Work out the finished part from the listing and answer in its coordinate system (mm). Face numbers are marked on the shaded views. Give positions to 0.01 mm unless a question says otherwise; leave off trailing zeros. Write each loop counter-clockwise with the first axis right and the second up, starting at its lowest first coordinate (ties: lowest second). Pieces come first, ordered by that corner, then holes. Notation, with made-up numbers: (52.25, 42.25) - (98.25, 42.25) arc R20 cw to (98.25, 55.25) - close; hole circle Ø10 at (46.5, 45). An arc over 180 degrees is marked (long way). Write item = value, one per line.
Autodesk Inventor part; units mm, degrees
ref_plane "YZ Plane" through (0, 0, 0) normal (1, 0, 0) x (0, 1, 0)
ref_plane "XZ Plane" through (0, 0, 0) normal (0, 1, 0) x (-1, 0, 0)
ref_plane "XY Plane" through (0, 0, 0) normal (0, 0, 1) x (1, 0, 0)
sketch "Sketch1" plane through (0, 0, 0) normal (0, 0, 1) x (1, 0, 0)
  line L0 (1.5875, 0) -> (1.5875, 8.89)
  line L1 (1.5875, 8.89) -> (2.4832, 3.81)
  line L2 (1.5875, 8.89) -> (6.7459, 8.89) construction
  line L3 (2.4832, 3.81) -> (2.085, 3.81)
  line L4 (2.085, 3.81) -> (2.4832, 1.5517)
  line L5 (2.4832, 1.5517) -> (1.8611, 1.5517)
  line L6 (1.8611, 1.5517) -> (1.8611, 0)
  line L7 (1.8611, 0) -> (1.5875, 0)
  line L8 (0, -4.826) -> (0, 11.176)
  line L9 (1.5875, 0) -> (1.8611, 0)
  line L10 (1.8611, 0) -> (1.8611, -2.54)
  line L11 (1.8611, -2.54) -> (1.5875, -2.54)
  line L12 (1.5875, -2.54) -> (1.5875, 0)
  point P0 (0, 0)
  point P1 (2.1722, 1.5517)
  dimension "d1" = 1.5875
  dimension "d3" = 0
  dimension "d4" = 80
  dimension "d5" = 0.3982
  dimension "d6" = 2.2583
  dimension "d7" = 1.5517
  dimension "d8" = 1.8611
  dimension "d10" = 8.89
  dimension "d11" = 2.54
  dimension "d12" = 0.2736
revolve "Revolution1" add sketch "Sketch1" angle 360 about axis through (0, -10, 0) along (0, 1, 0)
properties part number "eigthinch"
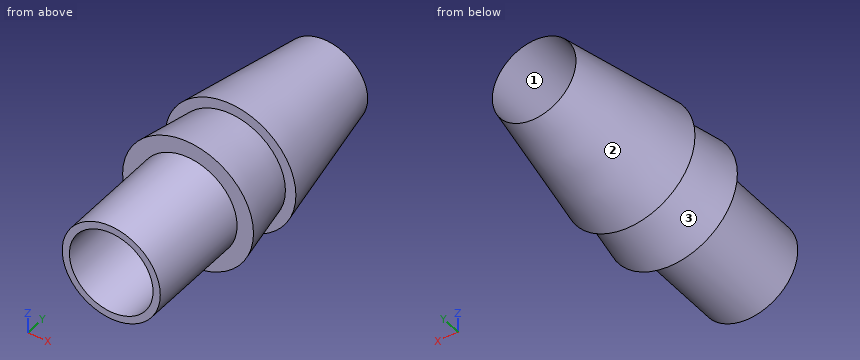
1. Find section D-D, the plane y = 6.75. Give the vertices of the cut face in (x, z) (1 decimal).
Solution:
outline = circle Ø3.9 at (0, 0); hole circle Ø3.2 at (0, 0)
2. Straight lines are drawn through the part: line 1 (X direction, y = 1, z = 0); line 2 (X direction, y = 2, z = 0); line 3 (Z direction, x = 0, y = 2.75). For each, find the intervals that lie inside material, in ascending order.
Solution:
line_1 = -1.86 to -1.59, 1.59 to 1.86
line_2 = -2.4 to -1.59, 1.59 to 2.4
line_3 = -2.27 to -1.59, 1.59 to 2.27
3. Find section C-C, the plane y = -0.5. Give the vertices of the cut face in (x, z) (1 decimal).
Solution:
outline = circle Ø3.7 at (0, 0); hole circle Ø3.2 at (0, 0)
4. For a pull along Y with two mould halves and no side action, classify the marked faces 1, 2 and 3 as pulls with the +Y half, pulls with the -Y half, needs draft (parallel to the pull), parting line crosses it, or undercut.
Solution:
face_1 = needs draft
face_2 = pulls with the +Y half
face_3 = undercut
5. Given pin 1 (2.5 mm diameter, centred on x = 0, z = 0, fed in from +Y); pin 2 (1 mm diameter, centred on y = -1, z = -1.5, fed in from -X), each flat-ended and moving along its own axis, determine where each tip first touches the part or whether it passes through.
Solution:
pin_1 = through
pin_2 = -1.57
